from build123d import *

# Parameters (mm, degrees)
ESBO_O1_R                  = 1.5
RESSALTO_EXTRUS_O1_DEPTH   = 20
RESSALTO_EXTRUS_O1_2_DEPTH = 20
RESSALTO_EXTRUS_O1_3_DEPTH = 20
RESSALTO_EXTRUS_O1_4_DEPTH = 20
ESBO_O2_W                  = 70
ESBO_O2_H                  = 150
RESSALTO_EXTRUS_O2_DEPTH   = 3


with BuildPart() as part:
    # Esbo_o1 → Ressalto-extrus_o1 (new body)
    with BuildSketch(Plane.XY):
        with Locations((33.5, 148)):
            Circle(ESBO_O1_R)
    extrude(amount=RESSALTO_EXTRUS_O1_DEPTH)



with BuildPart() as body_2:
    # Esbo_o1 → Ressalto-extrus_o1 2 (new body)
    with BuildSketch(Plane.XY):
        with Locations((-33.5, 148)):
            Circle(ESBO_O1_R)
    extrude(amount=RESSALTO_EXTRUS_O1_2_DEPTH)


with BuildPart() as body_3:
    # Esbo_o1 → Ressalto-extrus_o1 3 (new body)
    with BuildSketch(Plane.XY):
        with Locations((33.5, 2)):
            Circle(ESBO_O1_R)
    extrude(amount=RESSALTO_EXTRUS_O1_3_DEPTH)


with BuildPart() as body_4:
    # Esbo_o1 → Ressalto-extrus_o1 4 (new body)
    with BuildSketch(Plane.XY):
        with Locations((-33.5, 2)):
            Circle(ESBO_O1_R)
    extrude(amount=RESSALTO_EXTRUS_O1_4_DEPTH)


with BuildPart() as part_1:
    add(part.part)

    add(body_2.part)  # Ressalto-extrus_o2 merges body 2

    add(body_3.part)  # Ressalto-extrus_o2 merges body 3

    add(body_4.part)  # Ressalto-extrus_o2 merges body 4
    # Esbo_o2 → Ressalto-extrus_o2 (add)
    with BuildSketch(Plane.XY.offset(20)):
        with Locations((0, 75)):
            Rectangle(ESBO_O2_W, ESBO_O2_H)
    extrude(amount=RESSALTO_EXTRUS_O2_DEPTH)


solid = part_1.part
Check sheet for the modelled part. Datum: model origin and axes. Units: mm. A direction names the side the tool comes from. Round coordinates to 2 decimals unless told otherwise and drop trailing zeros. Order: outer loops, then holes, each group sorted by start corner. A loop starts at its lowest first (then second) coordinate and runs counter-clockwise, first axis right, second up. Notation, with made-up numbers: M -1,-32.75 L 7,-32.75 A17 ccw 7,-6.75 Z; hole C 77,-12.75 d6. An arc over 180 degrees is marked long. One line per item, written item: value. Start each with the question number.
1. Scan line: line 1 along Z through (x, y) = (8, 97.5). Record every from-to range of solid material in increasing order.
2. Section check B-B on x = -33.5. Enter the section's corners in (y, z).
3. Section check C-C on y = 130.5. Enter the section's corners in (x, z).
4. Release check for a two-part mould opening along X. For faces 1 (the flat face through (33, 2, 0)), 2 (the flat face through (-35, 74, 21)), 3 (the cylindrical face through (-33.695, 149.487, 9.86)) record: released by +X, released by -X, zero draft, split by the parting line, or undercut.
5. Section check D-D on x = 15. Enter the section's corners in (y, z), and give its area (3 significant figures).
6. Gauge pin test, flat end, axial feed: P1, Ø4, axis at x = 12, y = 68, coming from the -Z side. Record the tip position at first contact, or that the pin passes through.
7. Section check A-A on z = 8.75. Enter the section's corners in (x, y).
8. Access from +Z, -Z, +X, -X, +Y, -Y to the whole of each face (thin tool, end or side, straight path). Record for faces 4 (the flat face through (33, 148, 0)), 5 (the cylindrical face through (33.305, 149.487, 9.86)).
Results found:
1. line 1: 20 to 23
2. outline: M 0,20 L 0.5,20 L 0.5,0 L 3.5,0 L 3.5,20 L 146.5,20 L 146.5,0 L 149.5,0 L 149.5,20 L 150,20 L 150,23 L 0,23 Z
3. outline: M -35,20 L 35,20 L 35,23 L -35,23 Z
4. face 1: zero draft
4. face 2: released by -X
4. face 3: undercut
5. outline: M 0,20 L 150,20 L 150,23 L 0,23 Z
5. area: 450 mm^2
6. P1: z = 20
7. outline: C -33.5,2 d3; C -33.5,148 d3; C 33.5,2 d3; C 33.5,148 d3
8. face 4: -Z, +X, -X, +Y, -Y
8. face 5: -Z
